Source: CAD feature listing. Evaluate the final solid. Frame: model axes, mm. Face numbers are marked on the shaded views. A direction names the side the tool comes from. Coordinates: 2 decimals unless noted, no trailing zeros. Order: outer loops, then holes, each group sorted by start corner. A loop starts at its lowest first (then second) coordinate and runs counter-clockwise, first axis right, second up.
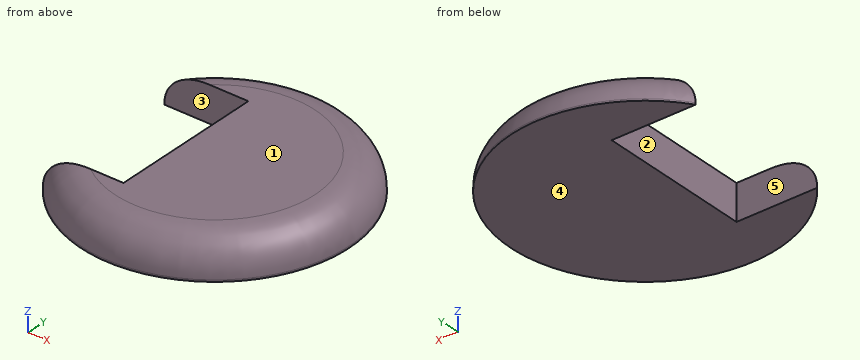
```python
from build123d import *

# Parameters (mm, degrees)
SKETCH037_R     = 7.5
PAD014_DEPTH    = 2
FILLET_R        = 1.9
SKETCH038_W     = 7.549545
SKETCH038_H     = 8.681977
POCKET016_DEPTH = 5


with BuildPart() as part:
    # Sketch037 → Pad014 (new body)
    with BuildSketch(Plane.XY):
        with Locations((102.610229, -47.581253)):
            Circle(SKETCH037_R)
    extrude(amount=PAD014_DEPTH)

    # Fillet
    fillet_edges = [part.edges().sort_by_distance(p)[0] for p in [
        (95.110229, -47.581253, 2),
    ]]
    fillet(fillet_edges, radius=FILLET_R)

    # Sketch038 (on Face4 of Fillet) → Pocket016 (cut)
    with BuildSketch(Plane.XY.offset(2)):
        with Locations((97.318771, -47.714951)):
            Rectangle(SKETCH038_W, SKETCH038_H)
    extrude(amount=-POCKET016_DEPTH, mode=Mode.SUBTRACT)


with BuildPart() as part_1:
    # Body006 placement: moved
    add(part.part.moved(Location((0, 0, 40))))


solid = part_1.part
```
1. Access query for the marked faces 1 and 2. Directions: +Z, -Z, +X, -X, +Y, -Y. A direction counts if a zero-diameter tool reaches every point of the face in a straight line with its end or side. Return the directions, or none.
Findings:
face 1: +Z, +X, -X, +Y, -Y
face 2: +Z, -Z, -X
2. Pin query (flat end, axial travel): P1, Ø1, axis at x = 98, z = 41, coming from the +Y side; P2, Ø1, axis at y = -44, z = 41, coming from the -X side. Return the tip coordinate at first contact, or that it passes through.
Findings:
P1: stops at y = -41.49
P2: stops at x = 101.09
3. Draft query along Y for the marked faces 3, 4 and 5. Return one class per face: released by +Y, released by -Y, zero draft, split by the parting line, or undercut.
Findings:
face 3: undercut
face 4: zero draft
face 5: undercut
4. Ray query, line 1 (Y direction, x = 100.5, z = 41); line 2 (X direction, y = -50.25, z = 41.1); line 3 (X direction, y = -43, z = 40.35). Return the intervals inside material, ascending.
Findings:
line 1: y = -54.54 to -52.06, -43.37 to -40.62
line 2: x = 101.09 to 109.31
line 3: x = 96.69 to 108.53
5. Section query A-A on z = 41.45. Return loops of the section in (x, y), plus the area to 3 significant figures.
Findings:
outline: (97.09, -43.37) - (101.09, -43.37) - (101.09, -52.06) - (97.31, -52.06) arc R6.94 ccw (long way) to start
area: 108 mm2
